Design review of the part built by this model. Coordinates are the model's own, in mm. A direction names the side the tool comes from. Coordinates: 2 decimals unless noted, no trailing zeros. Loops run counter-clockwise (first coordinate to the right, second up) from the corner with the lowest first, then second, coordinate; pieces in that order, holes last. Notation, with made-up numbers: (83.25, 83.25) -> (96.25, 83.25) arc R13 cw to (96.25, 108.25) -> close; hole circle Ø9 at (34.25, 32.5). An arc over 180 degrees is marked (long way). Use one line per item in the form item = value. Start each with the question number.
1. Machinability: for faces 1 (the face through (5, -2.5, 1)), 2 (the face through (16, 1.25, -4)), 3 (the face through (19.34, 1.05, 0.73)), which of the approach directions +Z, -Z, +X, -X, +Y, -Y give a long, thin tool a straight path to every point of the face, cutting with its end or side? Answer none if there is none.
2. The part is to be moulded in two halves that separate along Y. For faces 4 (the face through (18.5, 0, -4)), 5 (the face through (4, 0, 0)), 6 (the face through (-2, -2, 1)), 7 (the face through (13.5, 0, -4)), say which applies: released by +Y, released by -Y, zero draft, split by the parting line, or undercut.
3. For pin 1 (2 mm diameter, centred on y = -1.5, z = -3.5, fed in from -X); pin 2 (1.2 mm diameter, centred on y = 0.5, z = -3.5, fed in from -X); pin 3 (0.7 mm diameter, centred on x = 16.5, z = -3, fed in from +Y), all flat-tipped, find the tip position at first contact; note any pin that passes through.
4. Consider section D-D (x = 0). State the section outline as (y, z) points.
5. Consider section A-A (x = 16). State the section outline as (y, z) points, then the cut area to 3 significant figures.
6. Wall thickness on line 1 (X direction, y = 0, z = 1.55); line 2 (Y direction, x = 0, z = 1.55); line 3 (Z direction, x = -1.25, y = -2.25): over which ranges is each line inside the solid? List them lowest first. Write a range as from..to.
7. Consider section B-B (z = 1.5). State how many separate pieces and enclosed holes the cut face has, then the cut area to 3 significant figures.
8. Consider section C-C (z = -3.5). State the section outline as (x, y) points, then the cut area to 3 significant figures.
from build123d import *

# Parameters (mm, degrees)
F0_W      = 19
F0_H      = 5
F1_DEPTH  = 2
F4_ANGLE  = 180
F5_R      = 5.5
F6_DEPTH  = 2.5
F7_R      = 3.5
F8_DEPTH  = 2.5
F11_W     = 20
F11_H     = 5
F12_DEPTH = 12.5
F13_W     = 5
F13_H     = 2.5
F14_DEPTH = 25
F15_R     = 1
F16_DEPTH = 25
F17_R     = 2.49999


# Not quite as in the source:
# - a fillet or chamfer is up to 0.001 mm smaller than in the source, because OpenCascade refuses the exact size


with BuildPart() as f1:
    # F0 (on Top) → F1 (new body)
    with BuildSketch(Plane.XY):
        with Locations((6.5, 0)):
            Rectangle(F0_W, F0_H)
    extrude(amount=F1_DEPTH)



with BuildPart() as f4:
    # F3 (on offset) → F4 (revolve)
    with BuildSketch(Plane.XY.offset(-0.5)):
        with BuildLine():
            ThreePointArc((21.5, 0), (16, 5.5), (10.5, 0))
            Line((10.5, 0), (21.5, 0))
        make_face()
    revolve(axis=Axis((22.6478228122, 0, -0.5), (-1, 0, 0)), revolution_arc=F4_ANGLE)


with BuildPart() as f1_1:
    add(f1.part)

    add(f4.part)  # F6 merges F4
    # F5 (on offset) → F6 (join, through all)
    with BuildSketch(Plane.XY.offset(-0.5)):
        with Locations((16, 0)):
            Circle(F5_R)
    extrude(amount=F6_DEPTH)

    # F7 (on offset) → F8 (cut, through all)
    with BuildSketch(Plane.XY.offset(-0.5)):
        with Locations((16, 0)):
            Circle(F7_R)
    extrude(amount=F8_DEPTH, mode=Mode.SUBTRACT)

    # F9 (on offset) → F10 (revolve, cut)
    with BuildSketch(Plane.XY.offset(-0.5)):
        with BuildLine():
            ThreePointArc((12.5, 0), (16, -3.5), (19.5, 0))
            Line((19.5, 0), (12.5, 0))
        make_face()
    revolve(axis=Axis((18.6947258189, 0, -0.5), (1, 0, 0)), mode=Mode.SUBTRACT)

    # F11 (on Front) → F12 (cut, symmetric)
    with BuildSketch(Plane.XZ):
        with Locations((16, -7.5)):
            Rectangle(F11_W, F11_H)
    extrude(amount=F12_DEPTH, both=True, mode=Mode.SUBTRACT)

    # F13 (on Top) → F14 (cut)
    with BuildSketch(Plane.XY):
        with Locations((16, 0)):
            Rectangle(F13_W, F13_H)
    extrude(amount=-F14_DEPTH, mode=Mode.SUBTRACT)

    # F15 (on Top) → F16 (cut)
    with BuildSketch(Plane.XY):
        Circle(F15_R)
    extrude(amount=F16_DEPTH, mode=Mode.SUBTRACT)

    # F17 (radius 2.5 in the source; OpenCascade refuses exactly that, so slightly less here)
    f17_edges = [f1_1.edges().sort_by_distance(p)[0] for p in [
        (-3, -2.5, 1),
        (-3, 2.5, 1),
    ]]
    fillet(f17_edges, radius=F17_R)


solid = f1_1.part
Geometry check:
q1.face_1 = +Z, -Z, -X, -Y
q1.face_2 = +Z, -Z
q1.face_3 = +Z
q2.face_4 = undercut
q2.face_5 = zero draft
q2.face_6 = released by -Y
q2.face_7 = undercut
q3.pin_1 = 11.03
q3.pin_2 = 11.07
q3.pin_3 = 5.04
q4.outline = (-2.5, 0) -> (-1, 0) -> (-1, 2) -> (-2.5, 2) -> close; (1, 0) -> (2.5, 0) -> (2.5, 2) -> (1, 2) -> close
q5.outline = (-5.5, -0.5) arc R5.5 ccw to (-3.16, -5) -> (-1.25, -5) -> (-1.25, -3.77) arc R3.5 cw to (-3.5, -0.5) -> (-3.5, 2) -> (-5.5, 2) -> close; (1.25, -5) -> (3.16, -5) arc R5.5 ccw to (5.5, -0.5) -> (5.5, 2) -> (3.5, 2) -> (3.5, -0.5) arc R3.5 cw to (1.25, -3.77) -> close
q5.area = 31.3 mm²
q6.line_1 = -3..-1, 1..12.5, 19.5..21.5
q6.line_2 = -2.5..-1, 1..2.5
q6.line_3 = 0..2
q7.separate_pieces = 1
q7.enclosed_holes = 2
q7.area = 119 mm²
q8.outline = circle Ø9.22 at (16, 0); hole (13.5, -1.25) -> (14.7, -1.25) arc R1.8 ccw to (17.3, -1.25) -> (18.5, -1.25) -> (18.5, 1.25) -> (17.3, 1.25) arc R1.8 ccw to (14.7, 1.25) -> (13.5, 1.25) -> close
q8.area = 52.3 mm²
